```python
from build123d import *

# Parameters (mm, degrees)
F0_W     = 12.4
F0_H     = 5.8
F1_DEPTH = 7.9
F2_W     = 11.3
F2_H     = 5.5
F3_DEPTH = 30
F4_R     = 0.5
F5_W     = 3.6
F5_H     = 2.7
F6_DEPTH = 3
F7_W     = 0.7
F7_H     = 7.9
F8_DEPTH = 2


with BuildPart() as f1:
    # F0 (on Top) → F1 (new body)
    with BuildSketch(Plane.XY):
        Rectangle(F0_W, F0_H)
    extrude(amount=F1_DEPTH)

    # F2 (on face) → F3 (join)
    with BuildSketch(Plane(origin=(0, 0, 0), x_dir=(1, 0, 0), z_dir=(0, 0, -1))):
        Rectangle(F2_W, F2_H)
    extrude(amount=F3_DEPTH)

    # F4
    f4_edges = [f1.edges().sort_by_distance(p)[0] for p in [
        (-5.65, -2.75, -15),
        (5.65, -2.75, -15),
        (0, -2.75, -30),
        (5.65, 0, -30),
        (0, 2.75, -30),
        (-5.65, 0, -30),
        (5.65, 2.75, -15),
        (-5.65, 2.75, -15),
    ]]
    fillet(f4_edges, radius=F4_R)

    # F5 (on face) → F6 (join)
    with BuildSketch(Plane.XY.offset(7.9)):
        Rectangle(F5_W, F5_H)
    extrude(amount=F6_DEPTH)

    # F7 (on face) → F8 (join)
    with BuildSketch(Plane(origin=(0, 2.9, 0), x_dir=(-1, 0, 0), z_dir=(0, 1, 0))):
        with Locations((3.6, 3.95)):
            Rectangle(F7_W, F7_H)
        with Locations((-3.6, 3.95)):
            Rectangle(F7_W, F7_H)
    extrude(amount=F8_DEPTH)


solid = f1.part
```
Work out the finished part from the listing and answer in its coordinate system (mm). A direction names the side the tool comes from. Give positions to 0.01 mm unless a question says otherwise; leave off trailing zeros. Loops run counter-clockwise (first coordinate to the right, second up) from the corner with the lowest first, then second, coordinate; pieces in that order, holes last. Notation, with made-up numbers: (-39.5, 60.25) - (-1.5, 60.25) arc R23 cw to (-1.5, 80.25) - close; hole circle Ø4 at (-31, -4). An arc over 180 degrees is marked (long way). Use CSV: the item, a comma, the result in double quotes. Start each with the question number.
(1) Each of these flat-tipped pins is pushed along its axis until it touches: pin 1 (0.7 mm diameter, centred on x = -4.5, z = 5, fed in from +Y); pin 2 (2 mm diameter, centred on y = 4.5, z = 2, fed in from -X); pin 3 (4 mm diameter, centred on x = 4, y = -1.5, fed in from +Z). Where does it stop, or does it pass through?
(2) Find the intervals of material crossed by L1, parallel to X at y = 1.75, z = -8; L2, parallel to Y at x = 4.5, z = -12.5; L3, parallel to Z at x = 0.25, y = -2.25, in increasing order.
(3) A tool of negligible diameter and unlimited length cuts with its end or side. For faces 4 (the face through (5.65, 0, -15)), 5 (the face through (3.95, 4, 4)), 6 (the face through (0, 1.35, 9)), from which of +Z, -Z, +X, -X, +Y, -Y can it reach the whole face along a straight path? Write none if from no direction.
(4) Find section C-C, the plane x = 1. Determine the outline of the cut face in (y, z), plus the area to 3 significant figures.
(5) Determine the mould class of faces 1 (the face through (-3.95, 4, 4)), 2 (the face through (0, 2.75, -15)), 3 (the face through (-3.25, 4, 4)) for opening direction X: released by +X, released by -X, zero draft, split by the parting line, or undercut.
(6) Find section B-B, the plane z = -18. Determine the outline of the cut face in (x, y).
(7) Find section A-A, the plane y = 4.5. Determine the outline of the cut face in (x, z), plus the area to 3 significant figures.
(8) Find section D-D, the plane y = 1. Determine the outline of the cut face in (x, z), plus the area to 3 significant figures.
Results found:
1,pin 1,"y = 2.9"
1,pin 2,"x = -3.95"
1,pin 3,"z = 7.9"
2,L1,"-5.65 to 5.65"
2,L2,"-2.75 to 2.75"
2,L3,"-30 to 7.9"
3,face 4,"-Z, +X, +Y, -Y"
3,face 5,"+Z, -Z, +X, +Y"
3,face 6,"+Z, +X, -X, +Y"
4,outline,"(-2.9, 0) - (-2.75, 0) - (-2.75, -29.5) arc R0.5 ccw to (-2.25, -30) - (2.25, -30) arc R0.5 ccw to (2.75, -29.5) - (2.75, 0) - (2.9, 0) - (2.9, 7.9) - (1.35, 7.9) - (1.35, 10.9) - (-1.35, 10.9) - (-1.35, 7.9) - (-2.9, 7.9) - close"
4,area,"219 mm^2"
5,face 1,"released by -X"
5,face 2,"zero draft"
5,face 3,"undercut"
6,outline,"(-5.65, -2.25) arc R0.5 ccw to (-5.15, -2.75) - (5.15, -2.75) arc R0.5 ccw to (5.65, -2.25) - (5.65, 2.25) arc R0.5 ccw to (5.15, 2.75) - (-5.15, 2.75) arc R0.5 ccw to (-5.65, 2.25) - close"
7,outline,"(-3.95, 0) - (-3.25, 0) - (-3.25, 7.9) - (-3.95, 7.9) - close; (3.25, 0) - (3.95, 0) - (3.95, 7.9) - (3.25, 7.9) - close"
7,area,"11.1 mm^2"
8,outline,"(-6.2, 0) - (-5.65, 0) - (-5.65, -29.5) arc R0.5 ccw to (-5.15, -30) - (5.15, -30) arc R0.5 ccw to (5.65, -29.5) - (5.65, 0) - (6.2, 0) - (6.2, 7.9) - (1.8, 7.9) - (1.8, 10.9) - (-1.8, 10.9) - (-1.8, 7.9) - (-6.2, 7.9) - close"
8,area,"448 mm^2"
